```python
from build123d import *

# Parameters (mm, degrees)
F0_W      = 97
F0_H      = 97
F1_DEPTH  = 600
F2_W      = 97
F2_H      = 97
F3_DEPTH  = 48.5
F5_DEPTH  = 25
F7_DEPTH  = 25
F8_R      = 6
F9_DEPTH  = 72
F10_R     = 6
F11_DEPTH = 48.5
F12_R     = 6
F13_DEPTH = 72


with BuildPart() as f1:
    # F0 (on Front) → F1 (new body, symmetric)
    with BuildSketch(Plane.XZ):
        Rectangle(F0_W, F0_H)
    extrude(amount=F1_DEPTH, both=True)

    # F2 (on face) → F3 (cut)
    with BuildSketch(Plane.YZ.offset(48.5)):
        Rectangle(F2_W, F2_H)
    extrude(amount=-F3_DEPTH, mode=Mode.SUBTRACT)

    # F4 (on face) → F5 (cut)
    with BuildSketch(Plane.YZ.offset(48.5)):
        Polygon((-314.321284, 48.5), (-451.5, 48.5), (-548.5, -48.5), (-411.321284, -48.5), align=None)
    extrude(amount=-F5_DEPTH, mode=Mode.SUBTRACT)

    # F6 (on face) → F7 (cut)
    with BuildSketch(Plane(origin=(-48.5, 0, 0), x_dir=(0, -1, 0), z_dir=(-1, 0, 0))):
        Polygon((-324.220779, 48.5), (-451.5, 48.5), (-548.5, -48.5), (-421.220779, -48.5), align=None)
    extrude(amount=-F7_DEPTH, mode=Mode.SUBTRACT)

    # F8 (on face) → F9 (cut, through all)
    with BuildSketch(Plane.YZ.offset(23.5)):
        with Locations((-431.410642, 0)):
            Circle(F8_R)
    extrude(amount=-F9_DEPTH, mode=Mode.SUBTRACT)

    # F10 (on face) → F11 (cut, through all)
    with BuildSketch(Plane.YZ):
        Circle(F10_R)
    extrude(amount=-F11_DEPTH, mode=Mode.SUBTRACT)

    # F12 (on face) → F13 (cut, through all)
    with BuildSketch(Plane(origin=(-23.5, 0, 0), x_dir=(0, -1, 0), z_dir=(-1, 0, 0))):
        with Locations((-436.36039, 0)):
            Circle(F12_R)
    extrude(amount=-F13_DEPTH, mode=Mode.SUBTRACT)


solid = f1.part
```
Here's how the part is built. I have some questions about the finished solid (model axes, mm). A direction names the side the tool comes from. Give positions to 0.01 mm unless a question says otherwise; leave off trailing zeros. Loops run counter-clockwise (first coordinate to the right, second up) from the corner with the lowest first, then second, coordinate; pieces in that order, holes last. Notation, with made-up numbers: M 79,14 L 87,14 A25 cw 87,45 Z; hole C 22,80 d11. An arc over 180 degrees is marked long. Use one line per item in the form item = value. Start each with the question number.
Q1. If we section it at B-B (z = -27.5): Write out the boundary of the cut face in (x, y), then the cut area to 3 significant figures.
Q2. I need wall thicknesses on line 1 along Y through (x, z) = (-39, 1); line 2 along Y through (x, z) = (-18, -3); line 3 along Y through (x, z) = (35, 22.5). Which ranges of each line are inside material? Lowest first, please.
Q3. Which directions (+Z, -Z, +X, -X, +Y, -Y) give clear straight access to the entire face, cutting with the end or side of a thin tool? Please do faces 1 (the flat face through (36, -499, 1)), 2 (the flat face through (36.17, -363.5, -0.68)), 3 (the flat face through (-36.17, 373.4, -0.68)), 4 (the flat face through (-36, 499, 1)), 5 (the flat face through (23.5, -433, -10)).
Q4. If we section it at A-A (x = 38): Write out the boundary of the cut face in (y, z), then the cut area to 3 significant figures.
Q5. Thinking about a two-plate mould opening in Y: for faces 6 (the flat face through (-1, -600, 1)), 7 (the flat face through (48.5, -543, 10)), 8 (the flat face through (25, 48.5, -1)), which applies, +Y half, -Y half, draft (parallel to the pull), parting line (faces both ways), or undercut?
Q6. If we section it at C-C (y = -475): Write out the boundary of the cut face in (x, z).
Taken from the geometry:
q1.outline = M -48.5,-600 L 48.5,-600 L 48.5,-527.5 L 23.5,-527.5 L 23.5,-390.32 L 48.5,-390.32 L 48.5,-48.5 L 0,-48.5 L 0,48.5 L 48.5,48.5 L 48.5,600 L -48.5,600 L -48.5,527.5 L -23.5,527.5 L -23.5,400.22 L -48.5,400.22 Z
q1.area = 105,000 mm^2
q2.line_1 = -600 to -437.33, -425.49 to -5.92, 5.92 to 371.72, 499 to 600
q2.line_2 = -600 to -436.61, -426.21 to -5.2, 5.2 to 431.16, 441.56 to 600
q2.line_3 = -600 to -477.5, -340.32 to -48.5, 48.5 to 600
q3.face_1 = -Z, +X
q3.face_2 = +Z, +X
q3.face_3 = +Z, -X
q3.face_4 = -Z, -X
q3.face_5 = +X
q4.outline = M -600,-48.5 L -548.5,-48.5 L -451.5,48.5 L -600,48.5 Z; M -411.32,-48.5 L -48.5,-48.5 L -48.5,48.5 L -314.32,48.5 Z; M 48.5,-48.5 L 600,-48.5 L 600,48.5 L 48.5,48.5 Z; hole C 436.36,0 d12
q4.area = 93,600 mm^2
q5.face_6 = -Y half
q5.face_7 = draft
q5.face_8 = undercut
q6.outline = M -48.5,-48.5 L 23.5,-48.5 L 23.5,25 L 48.5,25 L 48.5,48.5 L -48.5,48.5 Z
